Verification items for the finished model (mm, model axes). Round coordinates to 2 decimals unless told otherwise and drop trailing zeros. Write each loop counter-clockwise with the first axis right and the second up, starting at its lowest first coordinate (ties: lowest second). Pieces come first, ordered by that corner, then holes. Notation, with made-up numbers: (87.25, 85.25) - (123.25, 85.25) arc R7 cw to (123.25, 95.25) - close; hole circle Ø1 at (-14, 39). An arc over 180 degrees is marked (long way). Answer as a JSON object with one key per item and string values.
```python
from build123d import *

# Parameters (mm, degrees)
SKETCH_1_R      = 1.5
EXTRUDE_1_DEPTH = 25
FILLET_1_R      = 10
FILLET_2_R      = 3


with BuildPart() as part:
    # 草图1 → 凸台-拉伸1 (new body)
    with BuildSketch(Plane.XY):
        Polygon((-17, 40), (17, 40), (17, 32), (25, 32), (25, -32), (17, -32), (17, -40), (-17, -40), (-17, -32), (-25, -32), (-25, 32), (-17, 32), align=None)
        with Locations((-13, 36)):
            Circle(SKETCH_1_R, mode=Mode.SUBTRACT)
        with Locations(Location((13, 36, 0), (0, 0, 180))):
            Circle(SKETCH_1_R, mode=Mode.SUBTRACT)
        with Locations(Location((-13, -36, 0), (0, 0, 180))):
            Circle(SKETCH_1_R, mode=Mode.SUBTRACT)
        with Locations((13, -36)):
            Circle(SKETCH_1_R, mode=Mode.SUBTRACT)
    extrude(amount=EXTRUDE_1_DEPTH)

    # 圆角1
    # the kernel refuses this fillet: 10 mm, written as the material it adds along each edge
    with BuildSketch(Plane(origin=(17, 32, 0), x_dir=(0, 1, 0), z_dir=(0, 0, 1)), Plane(origin=(-17, 32, 0), x_dir=(-1, 0, 0), z_dir=(0, 0, 1)), Plane(origin=(17, -32, 0), x_dir=(1, 0, 0), z_dir=(0, 0, 1)), Plane(origin=(-17, -32, 0), x_dir=(0, -1, 0), z_dir=(0, 0, 1))) as fillet_1_piece_1:
        with BuildLine():
            CenterArc((9.830951895, -9.830951895), FILLET_1_R, 100.550098012, 68.899803976)
            Line((0, -8), (0, 0))
            Line((0, 0), (8, 0))
        make_face()
    extrude(amount=25)

    # 圆角2
    fillet_2_edges = [part.edges().sort_by_distance(p)[0] for p in [
        (25, 32, 12.5),
        (25, -32, 12.5),
        (-25, -32, 12.5),
        (-25, 32, 12.5),
    ]]
    fillet(fillet_2_edges, radius=FILLET_2_R)


solid = part.part
```
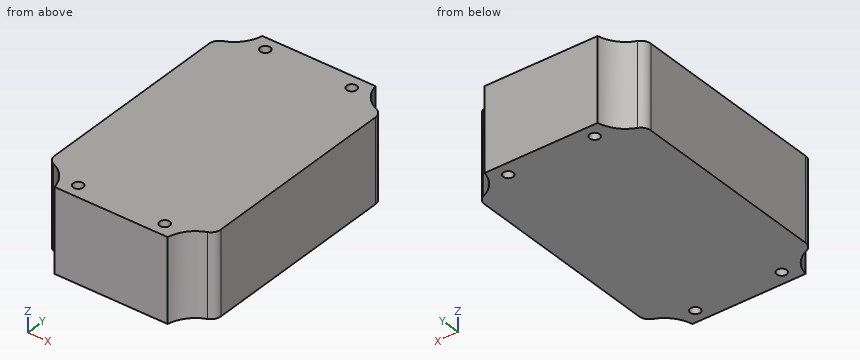
1. Go/stop test with a flat-tipped pin: pin 1 (5 mm diameter, centred on x = 13, y = -36, fed in from -Z). Record where the tip stops, or that it passes through.
Completed:
{"pin 1": "stops at z = 0"}
2. Cross-section at B-B (z = 19.75). Record the boundary of the cut face in (x, y), plus the area to 3 significant figures.
Completed:
{"outline": "(-25, -29.76) arc R3 ccw to (-23.11, -32.55) arc R10 cw to (-17, -40) - (17, -40) arc R10 cw to (23.11, -32.55) arc R3 ccw to (25, -29.76) - (25, 29.76) arc R3 ccw to (23.11, 32.55) arc R10 cw to (17, 40) - (-17, 40) arc R10 cw to (-23.11, 32.55) arc R3 ccw to (-25, 29.76) - close; hole circle Ø3 at (-13, -36); hole circle Ø3 at (-13, 36); hole circle Ø3 at (13, -36); hole circle Ø3 at (13, 36)", "area": "3,790 mm^2"}
3. Cross-section at A-A (x = 13). Record the boundary of the cut face in (y, z).
Completed:
{"outline": "(-40, 0) - (-37.5, 0) - (-37.5, 25) - (-40, 25) - close; (-34.5, 0) - (34.5, 0) - (34.5, 25) - (-34.5, 25) - close; (37.5, 0) - (40, 0) - (40, 25) - (37.5, 25) - close"}
4. Material ranges on probe 1 along Y at (x, z) = (-13, 18.5); probe 2 along Y at (x, z) = (23.5, 23.75), recorded low to high. Write a range as from..to.
Completed:
{"probe 1": "y = -40..-37.5, -34.5..34.5, 37.5..40", "probe 2": "y = -32.36..32.36"}
5. Cross-section at C-C (y = 36). Record the boundary of the cut face in (x, z), plus the area to 3 significant figures.
Completed:
{"outline": "(-18.71, 0) - (-14.5, 0) - (-14.5, 25) - (-18.71, 25) - close; (-11.5, 0) - (11.5, 0) - (11.5, 25) - (-11.5, 25) - close; (14.5, 0) - (18.71, 0) - (18.71, 25) - (14.5, 25) - close", "area": "785 mm^2"}
